Geometry: final body of the model. Coordinates: model frame, mm. A direction names the side the tool comes from. Give positions to 0.01 mm unless a question says otherwise; leave off trailing zeros. Write each loop counter-clockwise with the first axis right and the second up, starting at its lowest first coordinate (ties: lowest second). Pieces come first, ordered by that corner, then holes. Notation, with made-up numbers: (66, -8) -> (97, -8) arc R32 ccw to (97, 31) -> close; hole circle Ø3 at (88, -25). An arc over 180 degrees is marked (long way). Answer in a Markdown table with one row per item. Add a question column.
Autodesk Fusion 360 part; units mm, degrees
sketch "Sketch1" plane through (0, 0, 0) normal (0, 0, 1) x (1, 0, 0)
  line L0 (0, 0) -> (30, 0)
  line L1 (30, 0) -> (30, 50)
  line L2 (30, 50) -> (0, 50)
  line L3 (0, 50) -> (0, 0)
  dimension "d1" = 30
  dimension "d2" = 50
extrude "Extrude1" add sketch "Sketch1" along normal blind 5
sketch "Sketch3" plane through (30, 0, 0) normal (1, 0, 0) x (0, 1, 0)
  line L0 (0, 0) -> (50, 0)
  line L1 (50, 0) -> (50, 5)
  line L2 (50, 5) -> (0, 5)
  line L3 (0, 5) -> (0, 0)
  line L4 (50, 5) -> (10, 5)
  line L5 (10, 5) -> (10, 0)
  line L6 (10, 0) -> (50, 0)
  line L7 (50, 0) -> (50, 5)
  dimension "d9" = 40
  dimension "d10" = 5
extrude "Extrude3" add sketch "Sketch3" along normal blind 10 contours L0 L1 L2 L4 L5 L6 L7
sketch "Sketch4" plane through (0, 0, 0) normal (-1, 0, 0) x (0, -1, 0)
  line L0 (-50, 0) -> (0, 0)
  line L1 (0, 0) -> (0, 5)
  line L2 (0, 5) -> (-50, 5)
  line L3 (-50, 5) -> (-50, 0)
  line L4 (-50, 5) -> (-10, 5)
  line L5 (-10, 5) -> (-10, 0)
  line L6 (-10, 0) -> (-50, 0)
  line L7 (-50, 0) -> (-50, 5)
  dimension "d13" = 40
  dimension "d14" = 5
extrude "Extrude4" add sketch "Sketch4" along normal blind 10 contours L0 L2 L3 L4 L5 L6 L7
sketch "Sketch5" plane through (0, 0, 0) normal (-1, 0, 0) x (0, -1, 0)
  line L0 (-10, 5) -> (-10, 0)
  line L1 (-10, 0) -> (0, 0)
  line L2 (0, 0) -> (0, 5)
  line L3 (0, 5) -> (-10, 5)
  circle A0 centre (-2.5, 2.5) radius 2.5
  dimension "d17" = 5
extrude "Extrude5" add sketch "Sketch5" along normal blind 10 contours A0
sketch "Sketch6" plane through (30, 0, 0) normal (1, 0, 0) x (0, 1, 0)
  line L0 (10, 0) -> (10, 5)
  line L1 (10, 5) -> (0, 5)
  line L2 (0, 5) -> (0, 0)
  line L3 (0, 0) -> (10, 0)
  circle A0 centre (2.5, 2.5) radius 2.5
  dimension "d20" = 5
extrude "Extrude6" add sketch "Sketch6" along normal blind 10 contours A0
sketch "Sketch7" plane through (40, 0, 0) normal (1, 0, 0) x (0, 1, 0)
  line L0 (50, 0) -> (50, 5)
  line L1 (50, 5) -> (10, 5)
  line L2 (10, 5) -> (10, 0)
  line L3 (10, 0) -> (50, 0)
  circle A0 centre (47.5, 2.5) radius 2.5
  dimension "d23" = 5
extrude "Extrude7" add sketch "Sketch7" along normal blind 5 contours A0
sketch "Sketch8" plane through (-10, 0, 0) normal (-1, 0, 0) x (0, -1, 0)
  line L0 (-50, 0) -> (-10, 0)
  line L1 (-10, 0) -> (-10, 5)
  line L2 (-10, 5) -> (-50, 5)
  line L3 (-50, 5) -> (-50, 0)
  circle A0 centre (-47.5, 2.5) radius 2.5
  dimension "d26" = 5
extrude "Extrude8" add sketch "Sketch8" along normal blind 5 contours A0
Q1. Section A-A on x = -11. Return loops of the section in (y, z).
Q2. Line query: probe 1 along X at (y, z) = (7.5, 4.75); probe 2 along X at (y, z) = (14.5, 4.85); probe 3 along Y at (x, z) = (41, 2.3). Output: solid intervals per line, ascending. Write a range as from..to.
Q3. Contact query for flat-ended pins moving along their axis: pin 1 Ø1.5 at (y, z) = (13.5, 4) entering from -X; pin 2 Ø1.5 at (y, z) = (8, 1.5) entering from -X; pin 3 Ø1.2 at (y, z) = (1.5, 4) entering from +X; pin 4 Ø6 at (x, y) = (32.5, 22.5) entering from -Z. Output: stop coordinate, or through.
Q4. Section B-B on y = 43. Return loops of the section in (x, z), and give its area (3 significant figures).
Q5. Access query for faces 5 (the flat face through (35, 10, 3)), 6 (the flat face through (30, 0.5, 0.6)), 7 (the flat face through (30, 0.5, 4.4)). Directions: +Z, -Z, +X, -X, +Y, -Y. A direction counts if a zero-diameter tool reaches every point of the face in a straight line with its end or side. Return the directions, or none.
Q6. Pull-direction query (Y, two-part tool) for faces 1 (the flat face through (30, 7, 2)), 2 (the flat face through (-15, 48, 3)), 3 (the cylindrical face through (42.46, 49.81, 3.46)), 4 (the cylindrical face through (34.9, 0.5, 4)); classes: +Y half, -Y half, draft (parallel to the pull), parting line (faces both ways), or undercut.
Checks:
| question | item | result |
|---|---|---|
| 1 | outline | circle Ø5 at (47.5, 2.5) |
| 2 | probe 1 | 0..30 |
| 2 | probe 2 | -10..40 |
| 2 | probe 3 | 45.01..49.99 |
| 3 | pin 1 | x = -10 |
| 3 | pin 2 | x = 0 |
| 3 | pin 3 | x = 40 |
| 3 | pin 4 | z = 0 |
| 4 | outline | (-10, 0) -> (40, 0) -> (40, 5) -> (-10, 5) -> close |
| 4 | area | 250 mm^2 |
| 5 | face 5 | +Z, -Z, +X |
| 5 | face 6 | -Z, +X, -Y |
| 5 | face 7 | +Z, +X, -Y |
| 6 | face 1 | undercut |
| 6 | face 2 | draft |
| 6 | face 3 | parting line |
| 6 | face 4 | undercut |
